```python
from build123d import *

# Parameters (mm, degrees)
SKETCH3_R                       = 92.5
SKETCH3_R_2                     = 87.5
BOSS_EXTRUDE3_DEPTH             = 75
BOSS_EXTRUDE4_REACH             = 222.014
BOSS_EXTRUDE4_END_RADIUS        = 92.5
SKETCH4_W                       = 140
SKETCH4_H                       = 75
BOSS_EXTRUDE4_DIRECTION_2_DEPTH = 5


with BuildPart() as part:
    # Sketch3 → Boss-Extrude3 (new body)
    with BuildSketch(Plane.XY):
        Circle(SKETCH3_R)
        Circle(SKETCH3_R_2, mode=Mode.SUBTRACT)
    extrude(amount=BOSS_EXTRUDE3_DEPTH)

    # Boss-Extrude4: up to this cylinder (the profile starts outside it)
    boss_extrude4_end = Plane(origin=(0, 0, 37.5), z_dir=(0, 0, -1)) * Cylinder(BOSS_EXTRUDE4_END_RADIUS, 630.028, mode=Mode.PRIVATE)
    # Sketch4 → Boss-Extrude4 (add, up to the surface)
    with BuildSketch(Plane(origin=(0, 92.5, 0), x_dir=(1, 0, 0), z_dir=(0, 1, 0)), mode=Mode.PRIVATE) as boss_extrude4_sk1:
        with Locations((0, -37.5)):
            Rectangle(SKETCH4_W, SKETCH4_H)
    boss_extrude4_tool1 = extrude(boss_extrude4_sk1.sketch, amount=-BOSS_EXTRUDE4_REACH, mode=Mode.PRIVATE) - boss_extrude4_end
    add(boss_extrude4_tool1.solids().sort_by_distance((0, 92.5, 37.5))[0])
    add(boss_extrude4_tool1.solids().sort_by_distance((0, 92.5, 37.5))[1])

    # Sketch4 → Boss-Extrude4 direction 2 (add)
    with BuildSketch(Plane(origin=(0, 92.5, 0), x_dir=(1, 0, 0), z_dir=(0, 1, 0))):
        with Locations((0, -37.5)):
            Rectangle(SKETCH4_W, SKETCH4_H)
    extrude(amount=BOSS_EXTRUDE4_DIRECTION_2_DEPTH)


solid = part.part
```
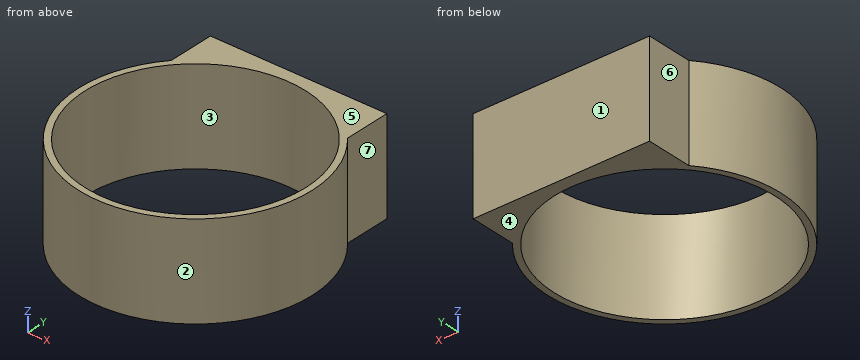
Part model, mm, in its own coordinate system. Face numbers are marked on the shaded views. A direction names the side the tool comes from. Round coordinates to 2 decimals unless told otherwise and drop trailing zeros. Order: outer loops, then holes, each group sorted by start corner. A loop starts at its lowest first (then second) coordinate and runs counter-clockwise, first axis right, second up. Notation, with made-up numbers: M -15,61 L 39,61 A23 cw 39,96 Z; hole C 76.25,22 d9. An arc over 180 degrees is marked long. Put each result on its own line as item: value. Start each with the question number.
1. Slice it at A-A on y = 0. List the corners of the cut face in (x, z).
2. Drill centre lines: probe 1 along Y at (x, z) = (0, 23); probe 2 along X at (y, z) = (1, 37.5); probe 3 along Y at (x, z) = (-16.5, 3). Where is each one in solid material? Low to high. Write a range as [from, to].
3. Tool access for the marked faces 5, 6 and 7: list every direction of +Z, -Z, +X, -X, +Y, -Y with a clear straight run to the whole face (end or side of a thin tool).
4. Two-plate mould, pull along Y, no slides. Class the marked faces 1, 2, 3 and 4: +Y half, -Y half, draft (parallel to the pull), parting line (faces both ways), or undercut.
5. Slice it at C-C on z = 34.5. List the corners of the cut face in (x, y), then the cut area to 3 significant figures.
6. Drop flat-ended pins along their axis: pin 1 (5 mm diameter, centred on y = -61.5, z = 14, fed in from -X); pin 2 (12 mm diameter, centred on y = -16, z = 9, fed in from -X); pin 3 (6 mm diameter, centred on y = 16, z = 14, fed in from +X). Give the stop position or say it passes through.
7. Slice it at B-B on x = 0. List the corners of the cut face in (y, z).
Findings:
1. outline: M -92.5,0 L -87.5,0 L -87.5,75 L -92.5,75 Z; M 87.5,0 L 92.5,0 L 92.5,75 L 87.5,75 Z
2. probe 1: [-92.5, -87.5], [87.5, 97.5]
2. probe 2: [-92.49, -87.49], [87.49, 92.49]
2. probe 3: [-91.02, -85.93], [85.93, 97.5]
3. face 5: +Z, +X, -X, +Y, -Y
3. face 6: +Z, -Z, -X, +Y
3. face 7: +Z, -Z, +X, +Y
4. face 1: +Y half
4. face 2: parting line
4. face 3: undercut
4. face 4: draft
5. outline: M -70,60.47 A92.5 ccw long 70,60.47 L 70,97.5 L -70,97.5 Z; hole C 0,0 d175
5. area: 4,900 mm2
6. pin 1: x = -71.24
6. pin 2: x = -91.96
6. pin 3: x = 91.58
7. outline: M -92.5,0 L -87.5,0 L -87.5,75 L -92.5,75 Z; M 87.5,0 L 97.5,0 L 97.5,75 L 87.5,75 Z
